CAD build for the part. Positions are in the model's coordinates, mm. Round coordinates to 2 decimals unless told otherwise and drop trailing zeros. Write each loop counter-clockwise with the first axis right and the second up, starting at its lowest first coordinate (ties: lowest second). Pieces come first, ordered by that corner, then holes. Notation, with made-up numbers: (46, 78) - (102, 78) arc R21 cw to (102, 113) - close; hole circle Ø6 at (86.25, 28). An arc over 180 degrees is marked (long way). Answer in a Markdown table with one row per item.
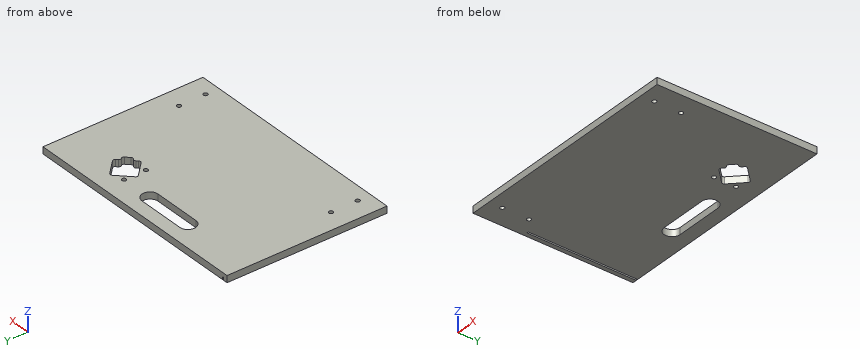
```python
from build123d import *

# Parameters (mm, degrees)
SKETCH1_W           = 438.1
SKETCH1_H           = 300
BOSS_EXTRUDE1_DEPTH = 12.7
CUT_EXTRUDE1_REACH  = 267.79
SKETCH2_R           = 4
FILLET1_R           = 4
SKETCH3_W           = 3.175
SKETCH3_H           = 205
CUT_EXTRUDE2_DEPTH  = 5
CUT_EXTRUDE3_REACH  = 267.79
SKETCH4_R           = 4
CUT_EXTRUDE4_REACH  = 267.79


with BuildPart() as part:
    # Sketch1 → Boss-Extrude1 (new body)
    with BuildSketch(Plane.XY):
        Rectangle(SKETCH1_W, SKETCH1_H)
    extrude(amount=BOSS_EXTRUDE1_DEPTH)

    # Sketch2 → Cut-Extrude1 (cut, up to next)
    with BuildSketch(Plane.XY.offset(12.7), mode=Mode.PRIVATE) as cut_extrude1_sk1:
        with Locations((76.214870385, 110.590065585)):
            Circle(SKETCH2_R)
    cut_extrude1_tool1 = extrude(cut_extrude1_sk1.sketch, amount=-CUT_EXTRUDE1_REACH, mode=Mode.PRIVATE) & part.part
    # Sketch2 → Cut-Extrude1 (cut, up to next)
    with BuildSketch(Plane.XY.offset(12.7), mode=Mode.PRIVATE) as cut_extrude1_sk2:
        with Locations((76.214870385, 69.409934415)):
            Circle(SKETCH2_R)
    cut_extrude1_tool2 = extrude(cut_extrude1_sk2.sketch, amount=-CUT_EXTRUDE1_REACH, mode=Mode.PRIVATE) & part.part
    # Sketch2 → Cut-Extrude1 (cut, up to next)
    with BuildSketch(Plane.XY.offset(12.7), mode=Mode.PRIVATE) as cut_extrude1_sk3:
        Polygon((99.05, 120.0520382), (68.9979618, 90), (99.05, 59.9479618), (107.71205807, 68.610019869), (113.368912319, 62.95316562), (126.09683438, 75.681087681), (120.439980131, 81.33794193), (129.1020382, 90), align=None)
    cut_extrude1_tool3 = extrude(cut_extrude1_sk3.sketch, amount=-CUT_EXTRUDE1_REACH, mode=Mode.PRIVATE) & part.part
    add(cut_extrude1_tool1.solids().sort_by_distance((76.21487, 110.590066, 12.7))[0], mode=Mode.SUBTRACT)
    add(cut_extrude1_tool2.solids().sort_by_distance((76.21487, 69.409934, 12.7))[0], mode=Mode.SUBTRACT)
    add(cut_extrude1_tool3.solids().sort_by_distance((100.368313, 88.681687, 12.7))[0], mode=Mode.SUBTRACT)

    # Fillet1
    fillet1_edges = [part.edges().sort_by_distance(p)[0] for p in [
        (99.05, 120.0520382, 6.35),
        (68.9979618, 90, 6.35),
        (120.439980131, 81.33794193, 6.35),
        (126.09683438, 75.681087681, 6.35),
        (113.368912319, 62.95316562, 6.35),
        (107.71205807, 68.610019869, 6.35),
        (99.05, 59.9479618, 6.35),
        (129.1020382, 90, 6.35),
    ]]
    fillet(fillet1_edges, radius=FILLET1_R - 0.0001)  # a hair under: the kernel refuses the full size

    # Sketch3 → Cut-Extrude2 (cut)
    with BuildSketch(Plane(origin=(0, 0, 0), x_dir=(-1, 0, 0), z_dir=(0, 0, -1))):
        with Locations((209.525, 47.5)):
            Rectangle(SKETCH3_W, SKETCH3_H)
    extrude(amount=-CUT_EXTRUDE2_DEPTH, mode=Mode.SUBTRACT)

    # Sketch4 → Cut-Extrude3 (cut, up to next)
    with BuildSketch(Plane(origin=(0, 0, 0), x_dir=(-1, 0, 0), z_dir=(0, 0, -1)), mode=Mode.PRIVATE) as cut_extrude3_sk1:
        with Locations((-180.95, -75)):
            Circle(SKETCH4_R)
    cut_extrude3_tool1 = extrude(cut_extrude3_sk1.sketch, amount=-CUT_EXTRUDE3_REACH, mode=Mode.PRIVATE) & part.part
    # Sketch4 → Cut-Extrude3 (cut, up to next)
    with BuildSketch(Plane(origin=(0, 0, 0), x_dir=(-1, 0, 0), z_dir=(0, 0, -1)), mode=Mode.PRIVATE) as cut_extrude3_sk2:
        with Locations(Location((-180.95, -125, 0), (0, 0, 180))):
            Circle(SKETCH4_R)
    cut_extrude3_tool2 = extrude(cut_extrude3_sk2.sketch, amount=-CUT_EXTRUDE3_REACH, mode=Mode.PRIVATE) & part.part
    # Sketch4 → Cut-Extrude3 (cut, up to next)
    with BuildSketch(Plane(origin=(0, 0, 0), x_dir=(-1, 0, 0), z_dir=(0, 0, -1)), mode=Mode.PRIVATE) as cut_extrude3_sk3:
        with Locations((180.95, -125)):
            Circle(SKETCH4_R)
    cut_extrude3_tool3 = extrude(cut_extrude3_sk3.sketch, amount=-CUT_EXTRUDE3_REACH, mode=Mode.PRIVATE) & part.part
    # Sketch4 → Cut-Extrude3 (cut, up to next)
    with BuildSketch(Plane(origin=(0, 0, 0), x_dir=(-1, 0, 0), z_dir=(0, 0, -1)), mode=Mode.PRIVATE) as cut_extrude3_sk4:
        with Locations(Location((180.95, -75, 0), (0, 0, 180))):
            Circle(SKETCH4_R)
    cut_extrude3_tool4 = extrude(cut_extrude3_sk4.sketch, amount=-CUT_EXTRUDE3_REACH, mode=Mode.PRIVATE) & part.part
    add(cut_extrude3_tool1.solids().sort_by_distance((180.95, -75, 0))[0], mode=Mode.SUBTRACT)
    add(cut_extrude3_tool2.solids().sort_by_distance((180.95, -125, 0))[0], mode=Mode.SUBTRACT)
    add(cut_extrude3_tool3.solids().sort_by_distance((-180.95, -125, 0))[0], mode=Mode.SUBTRACT)
    add(cut_extrude3_tool4.solids().sort_by_distance((-180.95, -75, 0))[0], mode=Mode.SUBTRACT)

    # Sketch5 → Cut-Extrude4 (cut, up to next)
    with BuildSketch(Plane.XY.offset(12.7), mode=Mode.PRIVATE) as cut_extrude4_sk1:
        with BuildLine():
            Line((15, 95), (-75, 95))
            ThreePointArc((-75, 95), (-90, 110), (-75, 125))
            Line((-75, 125), (15, 125))
            ThreePointArc((15, 125), (30, 110), (15, 95))
        make_face()
    cut_extrude4_tool1 = extrude(cut_extrude4_sk1.sketch, amount=-CUT_EXTRUDE4_REACH, mode=Mode.PRIVATE) & part.part
    add(cut_extrude4_tool1.solids().sort_by_distance((-30, 110, 12.7))[0], mode=Mode.SUBTRACT)


solid = part.part
```
Q1. Drill centre lines: line 1 (Y direction, x = -180.95, z = 3.75); line 2 (Y direction, x = -39, z = 3); line 3 (X direction, y = -36, z = 2.75). Where is each one in solid material? Low to high.
Computed:
| item | result |
|---|---|
| line 1 | y = -150 to -129, -121 to -79, -71 to 150 |
| line 2 | y = -150 to 95, 125 to 150 |
| line 3 | x = -219.05 to -211.11, -207.94 to 219.05 |
Q2. Flat gauge pins, fed straight in: pin 1 (3.5 mm diameter, centred on x = -209.5, y = 12, fed in from -Z); pin 2 (1 mm diameter, centred on x = -210, z = 2, fed in from +Y). Where does each tip first touch, or does it go through?
Computed:
| item | result |
|---|---|
| pin 1 | stops at z = 0 |
| pin 2 | stops at y = -55 |
Q3. Saw through at B-B on z = 7.5. Count the separate pieces of the cut face and the enclosed holes in it, then the cut area to 3 significant figures.
Computed:
| item | result |
|---|---|
| separate pieces | 1 |
| enclosed holes | 8 |
| area | 126,000 mm2 |
Q4. Saw through at A-A on x = -19.5. List the corners of the cut face in (y, z), then the cut area to 3 significant figures.
Computed:
| item | result |
|---|---|
| outline | (-150, 0) - (95, 0) - (95, 12.7) - (-150, 12.7) - close; (125, 0) - (150, 0) - (150, 12.7) - (125, 12.7) - close |
| area | 3,430 mm2 |
